from build123d import *

# Parameters (mm, degrees)
SALIENTE_EXTRUIR2_DEPTH = 0.4


with BuildPart() as part:
    # Croquis1 → Revolución1 (revolve)
    with BuildSketch(Plane.XY):
        Polygon((-10.9, 20), (-10.9, 0), (-12.25, 0), (-12.25, 18), (-22.25, 18), (-12.25, 20), align=None)
    revolve(axis=Axis((0, 0, 0), (0, 1, 0)))

    # Croquis3 → Saliente-Extruir2 (add)
    with BuildSketch(Plane(origin=(0, 20, 0), x_dir=(1, 0, 0), z_dir=(0, 1, 0))):
        with BuildLine():
            ThreePointArc((10.9, 0), (7.707463915, -7.707463915), (0, -10.9))
            ThreePointArc((0, -10.9), (-7.707463915, -7.707463915), (-10.9, 0))
            ThreePointArc((-10.9, 0), (-7.707463915, 7.707463915), (0, 10.9))
            ThreePointArc((0, 10.9), (7.707463915, 7.707463915), (10.9, 0))
        make_face()
        with BuildLine():
            Line((0.181294315, -2.493417809), (0, -10.639817501))
            Line((0, -10.639817501), (-0.181294315, -2.493417809))
            ThreePointArc((-0.181294315, -2.493417809), (-1.767766953, -1.767766953), (-2.493417809, -0.181294315))
            Line((-2.493417809, -0.181294315), (-10.639817501, 0))
            Line((-10.639817501, 0), (-2.493417809, 0.181294315))
            ThreePointArc((-2.493417809, 0.181294315), (-1.767766953, 1.767766953), (-0.181294315, 2.493417809))
            Line((-0.181294315, 2.493417809), (0, 10.639817501))
            Line((0, 10.639817501), (0.181294315, 2.493417809))
            ThreePointArc((0.181294315, 2.493417809), (1.767766953, 1.767766953), (2.493417809, 0.181294315))
            Line((2.493417809, 0.181294315), (10.639817501, 0))
            Line((10.639817501, 0), (2.493417809, -0.181294315))
            ThreePointArc((2.493417809, -0.181294315), (1.767766953, -1.767766953), (0.181294315, -2.493417809))
        make_face(mode=Mode.SUBTRACT)
    extrude(amount=-SALIENTE_EXTRUIR2_DEPTH)


solid = part.part
For this review, take the finished solid that the model builds, in its own axes (mm). A direction names the side the tool comes from. Coordinates: 2 decimals unless noted, no trailing zeros. Loops run counter-clockwise (first coordinate to the right, second up) from the corner with the lowest first, then second, coordinate; pieces in that order, holes last. Notation, with made-up numbers: (63, -22) -> (89, -22) arc R37 ccw to (89, 15) -> close; hole circle Ø8 at (-25.5, -22.5). An arc over 180 degrees is marked (long way). Write each question's results on one line, items separated by ' | '.
Q1. To check wall thickness, follow line 1 along Z through (x, y) = (0, 5.5); line 2 along Z through (x, y) = (10, 10.25); line 3 along X through (y, z) = (4.5, -3.5). State the ranges of each line that lie inside material, in increasing order. Write a range as [from, to].
Taken from the geometry:
line 1: [-12.25, -10.9], [10.9, 12.25] | line 2: [-7.08, -4.34], [4.34, 7.08] | line 3: [-11.74, -10.32], [10.32, 11.74]
Q2. For pin 1 Ø13 at (x, z) = (0, 0) entering from -Y; pin 2 Ø1 at (x, z) = (4, -15) entering from +Y; pin 3 Ø2 at (y, z) = (7.5, 1.5) entering from -X, all flat-tipped, find the tip position at first contact; note any pin that passes through.
Taken from the geometry:
pin 1: y = 19.6 | pin 2: y = 19.45 | pin 3: x = -12.24
Q3. Add section A-A, the plane y = 5. State the section outline as (x, z) points.
Taken from the geometry:
outline: circle Ø24.5 at (0, 0); hole circle Ø21.8 at (0, 0)
Q4. Machinability: for faces 1 (the flat face through (-3, 20, 3)), 2 (the flat face through (-2, 19.6, 2)), 3 (the cylindrical face through (1.75, 19.803, -1.785)), which of the approach directions +Z, -Z, +X, -X, +Y, -Y give a long, thin tool a straight path to every point of the face, cutting with its end or side? Answer none if there is none.
Taken from the geometry:
face 1: +Z, -Z, +X, -X, +Y | face 2: -Y | face 3: +Y, -Y
Q5. Mouldability with a two-part tool opening along Z and no side actions: class faces 4 (the cylindrical face through (1.785, 19.803, 1.75)), 5 (the flat face through (-11, 0, -2)), 6 (the cylindrical face through (-10.4, 9.66, 3.27)), 7 (the cylindrical face through (-6.586, 9.126, 10.329)) as +Z half, -Z half, draft (parallel to the pull), parting line (faces both ways), or undercut.
Taken from the geometry:
face 4: undercut | face 5: draft | face 6: undercut | face 7: parting line
